Build history of the part. All positions in model axes, mm. A direction names the side the tool comes from. Give positions to 0.01 mm unless a question says otherwise; leave off trailing zeros. Loops run counter-clockwise (first coordinate to the right, second up) from the corner with the lowest first, then second, coordinate; pieces in that order, holes last. Notation, with made-up numbers: (-38.75, -18.75) -> (-22.75, -18.75) arc R7 ccw to (-22.75, -9.75) -> close; hole circle Ø7 at (-33, -40). An arc over 180 degrees is marked (long way). Answer as a JSON object with one key per item and string values. Group by question number.
Q1. Two-plate mould, pull along X, no slides. Class faces 1 (the flat face through (24, 0, -7)), 2 (the cylindrical face through (8.23, -14.3, -36.89)), 3 (the flat face through (19, -1.5, -37)), 4 (the flat face through (7.99, 16.84, -36.91)): pulls with the +X half, pulls with the -X half, needs draft (parallel to the pull), parting line crosses it, or undercut.
Q2. Drop flat-ended pins along their axis: pin 1 (3 mm diameter, centred on x = -17.5, z = -38, fed in from +Y); pin 2 (2 mm diameter, centred on x = 20.5, y = 15.5, fed in from +Z); pin 3 (2 mm diameter, centred on y = 6.5, z = -2.5, fed in from -X). Give the stop position or say it passes through.
Q3. Tool access for faces 5 (the flat face through (7.99, -16.84, -36.91)), 6 (the flat face through (27, 6, -3)), 7 (the conical face through (-0.49, 25.4, -7.87)), 8 (the cylindrical face through (-16.5, 0, -36.9)): list every direction of +Z, -Z, +X, -X, +Y, -Y with a clear straight run to the whole face (end or side of a thin tool).
Q4. Wall check: probe 1 along X at (y, z) = (-6, 34.5); probe 2 along X at (y, z) = (0, 16.5); probe 3 along Z at (x, y) = (2.5, 5). Give the ranges that are in metal, low to high. Write a range as from..to.
Q5. Band-saw the part on D-D, the plane z = 22.5. Write the cut outline in (x, y), plus the area to 3 significant figures.
Q6. Band-saw the part on C-C, the plane z = -33. Write the cut outline in (x, y), plus the area to 3 significant figures.
from build123d import *

# Parameters (mm, degrees)
F0_W            = 25
F0_H            = 4.9944465005
F0_W_2          = 20
F0_H_2          = 20
F2_SIZE         = 2
F5_DEPTH        = 63.5294467211
F7_R            = 7.5
F8_DEPTH        = 1.5
F8_COPIES_COUNT = 6
F9_R            = 8.5
F10_DEPTH       = 89.8396968842


# Not quite as in the source:
# - a pattern or mirror of a feature is missing from the dataset's text; its kind, count and spacing are read off the source's solid


with BuildPart() as f1:
    # F0 (on Front) → F1 (revolve)
    with BuildSketch(Plane.XZ):
        Polygon((0, 40), (0, 0), (22.225, 0), (22.225, 2), (11.1490100557, 40), align=None)
        Polygon((22.225, 0), (0, 0), (0, -4.35), (31.5, -4.35), (31.5, 0), align=None)
        Polygon((31.5, -4.35), (0, -4.35), (0, -8.1027767497), (25, -8.1027767497), align=None)
        with Locations((12.5, -10.6)):
            Rectangle(F0_W, F0_H)
        Polygon((25, -13.0972232503), (0, -13.0972232503), (0, -16.85), (31.5, -16.85), align=None)
        Polygon((31.5, -16.85), (0, -16.85), (0, -27), (20, -27), (31.5, -27), align=None)
        with Locations((10, -37)):
            Rectangle(F0_W_2, F0_H_2)
    revolve(axis=Axis((0, 0, -0.6091467625), (0, 0, -1)))

    # F2
    f2_edges = [f1.edges().sort_by_distance(p)[0] for p in [
        (-31.5, 0, -27),
        (-20, 0, -47),
    ]]
    chamfer(f2_edges, length=F2_SIZE)

    # F4 (on offset) → F5 (cut)
    with BuildSketch(Plane.YZ.offset(24)):
        with BuildLine():
            ThreePointArc((-6, -8.1027767497), (0, -14.1027767497), (6, -8.1027767497))
            ThreePointArc((6, -8.1027767497), (0, -2.1027767497), (-6, -8.1027767497))
        make_face()
        with BuildLine():
            ThreePointArc((-6, -8.1027767497), (0, -2.1027767497), (6, -8.1027767497))
            Line((6, -8.1027767497), (6, 0))
            Line((6, 0), (-6, 0))
            Line((-6, 0), (-6, -8.1027767497))
        make_face()
    extrude(amount=F5_DEPTH, mode=Mode.SUBTRACT)

    # F6: F1 across plane


with BuildPart() as f1_1:
    add(f1.part)
    add(f1.part.mirror(Plane.YZ), mode=Mode.INTERSECT)

    # F7 (on Front) → F8 (cut, symmetric)
    with BuildSketch(Plane.XZ):
        with Locations((24, -37)):
            Circle(F7_R)
    f8 = extrude(amount=F8_DEPTH, both=True, mode=Mode.SUBTRACT)

    # F8_copies: F8 ×6 about axis
    f8_copies_axis = Axis((0, 0, 0), (0, 0, 1))
    for i in range(1, F8_COPIES_COUNT):
        add(f8.rotate(f8_copies_axis, i * 360 / F8_COPIES_COUNT), mode=Mode.SUBTRACT)

    # F9 (on Top) → F10 (cut)
    with BuildSketch(Plane.XY):
        Circle(F9_R)
    extrude(amount=F10_DEPTH, mode=Mode.SUBTRACT)


solid = f1_1.part
Worked answers:
{
 "1": {"face 1": "pulls with the +X half", "face 2": "undercut", "face 3": "needs draft", "face 4": "undercut"},
 "2": {"pin 1": "y = 12", "pin 2": "z = 0", "pin 3": "x = -30.92"},
 "3": {"face 5": "none", "face 6": "+Z, +X", "face 7": "+Y", "face 8": "-X"},
 "4": {"probe 1": "-11.25..-6.02, 6.02..11.25", "probe 2": "-18..-8.5, 8.5..18", "probe 3": "-47..0"},
 "5": {"outline": "circle Ø32.5 at (0, 0); hole circle Ø17 at (0, 0)", "area": "603 mm2"},
 "6": {"outline": "(-19.94, -1.5) arc R20 ccw to (-11.27, -16.52) -> (-10.13, -14.54) -> (-7.53, -16.04) -> (-8.67, -18.02) arc R20 ccw to (8.67, -18.02) -> (7.53, -16.04) -> (10.13, -14.54) -> (11.27, -16.52) arc R20 ccw to (19.94, -1.5) -> (17.66, -1.5) -> (17.66, 1.5) -> (19.94, 1.5) arc R20 ccw to (11.27, 16.52) -> (10.13, 14.54) -> (7.53, 16.04) -> (8.67, 18.02) arc R20 ccw to (-8.67, 18.02) -> (-7.53, 16.04) -> (-10.13, 14.54) -> (-11.27, 16.52) arc R20 ccw to (-19.94, 1.5) -> (-17.66, 1.5) -> (-17.66, -1.5) -> close", "area": "1,210 mm2"}
}
